Input: part model. Units: mm. Frame: model coordinates. Face numbers are marked on the shaded views. A direction names the side the tool comes from. Round coordinates to 2 decimals unless told otherwise and drop trailing zeros. Loops run counter-clockwise (first coordinate to the right, second up) from the corner with the lowest first, then second, coordinate; pieces in that order, holes last. Notation, with made-up numbers: (40, -25) - (54, -25) arc R9 cw to (54, -9) - close; hole circle Ø5 at (3, 75). An arc over 180 degrees is marked (long way). One line per question, with ' | ' between items. Start each with the question number.
Item 1: Set-up query: the marked faces 1, 2, 3 and 4. Return all of +Z, -Z, +X, -X, +Y, -Y with unobstructed straight access to the full face (end or side cutting, diameter ignored); none if empty.
Item 2: First-contact query: pin 1 (3 mm diameter, centred on x = -93, y = 44, fed in from -Z); pin 2 (7 mm diameter, centred on y = -10, z = 45, fed in from -X); pin 3 (5 mm diameter, centred on x = -86, z = 46.5, fed in from -Y). Flat tips, straight axial feed; report the tip coordinate or a pass-through.
Item 3: Section B-B, the plane y = 38. Return loops of the section in (x, z).
Item 4: Material intervals for line 1 along Z through (x, y) = (-20, -10); line 2 along Z through (x, y) = (-12.5, 12); line 3 along Y through (x, z) = (-29.25, 45), sorted ascending.
Item 5: Section C-C, the plane z = 45. Return loops of the section in (x, y).
Item 6: Section D-D, the plane x = -14. Return loops of the section in (y, z).
Item 7: Section A-A, the plane z = 75. Return loops of the section in (x, y), plus the area to 3 significant figures.
Autodesk Fusion 360 part; units mm, degrees
sketch "Sketch3" plane through (0, 0, 0) normal (0, 0, 1) x (1, 0, 0)
  line L0 (0, 0) -> (-40, 0)
  line L1 (-40, 0) -> (-40, 60)
  line L2 (-40, 60) -> (0, 60)
  line L3 (0, 60) -> (0, 0)
  line L4 (-17.9857, 0) -> (-23.9857, 0)
  line L5 (-23.9857, 0) -> (-23.9857, -20)
  line L6 (-23.9857, -20) -> (-17.9857, -20)
  line L7 (-17.9857, -20) -> (-17.9857, 0)
  line L8 (-40, 0) -> (-23.9857, -20)
  line L9 (-17.9857, 0) -> (2.0143, 0)
  line L10 (2.0143, 0) -> (2.0143, 1.9843)
  line L11 (2.0143, 1.9843) -> (2.0143, 60)
  line L12 (2.0143, 60) -> (0, 60)
  dimension "d16" = 60
  dimension "d17" = 40
  dimension "d18" = 20
  dimension "d19" = 6
  dimension "d63" = 20
extrude "Extrude1" add sketch "Sketch3" along normal blind 85 contours L0 L1 L2 L3 L4 L9 | L0 L4 L5 L6 L7 | L0 L5 L8
sketch "Sketch5" plane through (0, 0, 85) normal (0, 0, 1) x (-1, 0, 0)
  line L0 (23.9857, 20) -> (17.9857, 20)
  line L1 (17.9857, 20) -> (17.9857, 0)
  line L2 (17.9857, 0) -> (0, 0)
  line L3 (0, 0) -> (0, -60)
  line L4 (0, -60) -> (40, -60)
  line L5 (40, -60) -> (40, 0)
  line L6 (40, -60) -> (0, -60)
  line L7 (0, -6) -> (23.9857, -6)
  line L8 (23.9857, -6) -> (23.9857, 0)
  line L9 (40, 0) -> (23.9857, 20)
  line L10 (23.9857, 0) -> (23.9857, 20)
  dimension "d20" = 6
extrude "Extrude2" cut sketch "Sketch5" against normal blind 15 contours L3 L4 L5 L6 L7 L8 L9 L10
sketch "Sketch6" plane through (-40, 0, 0) normal (-1, 0, 0) x (0, -1, 0)
  line L0 (0, 70) -> (-60, 70)
  line L1 (-60, 70) -> (-60, 0)
  line L2 (-60, 0) -> (0, 0)
  line L3 (-55, 0) -> (-10, 0)
  line L4 (-10, 0) -> (-10, 60)
  line L5 (-10, 60) -> (-55, 60)
  line L6 (-55, 60) -> (-55, 0)
  line L7 (0, 0) -> (0, 70)
  dimension "d23" = 45
  dimension "d27" = 10
  dimension "d28" = 60
extrude "Extrude3" cut sketch "Sketch6" against normal blind 30 contours L2 L3 L4 L5 L6
sketch "Sketch7" plane through (0, 60, 0) normal (0, 1, 0) x (-1, 0, 0)
  line L0 (40, 70) -> (0, 70)
  line L1 (0, 70) -> (0, 0)
  line L2 (0, 0) -> (40, 0)
  line L3 (40, 0) -> (40, 70)
  line L4 (20, 70) -> (20, 10) construction
  circle A0 centre (20, 10) radius 2
  point P0 (20, 10)
  dimension "d29" = 60
  dimension "d30" = 20
  dimension "d31" = 4
extrude "Extrude4" cut sketch "Sketch7" against normal blind 57 contours A0
sketch "Sketch8" plane through (0, 55, 0) normal (0, -1, 0) x (1, 0, 0)
  circle A0 centre (-20, 10) radius 2
  line L0 (-40, 60) -> (-40, 0)
  line L1 (-40, 0) -> (-10, 0)
  line L2 (-10, 0) -> (-10, 60)
  line L3 (-10, 60) -> (-40, 60)
  line L4 (-10, 0) -> (-25, 0)
  line L5 (-25, 0) -> (-25, 10)
  line L6 (-20, 15) -> (-10, 15)
  line L7 (-10, 15) -> (-10, 0)
  arc A1 (-20, 15) -> (-25, 10) centre (-20, 10) ccw
  dimension "d34" = 5
extrude "Extrude5" add sketch "Sketch8" along normal blind 19 contours L1 L2 L4 L5 L6 L7 A1
sketch "Sketch10" plane through (0, 36, 0) normal (0, -1, 0) x (1, 0, 0)
  circle A0 centre (-20, 10) radius 2
  line L0 (-10, 15) -> (-20, 15)
  arc A1 (-20, 15) -> (-25, 10) centre (-20, 10) ccw
  line L1 (-25, 10) -> (-25, 0)
  line L2 (-25, 0) -> (-10, 0)
  line L3 (-10, 0) -> (-10, 15)
  line L4 (-20, 10) -> (-90.5618, 57.3923)
  dimension "d39" = 85
sketch "Sketch11" plane through (-40, 0, 0) normal (-1, 0, 0) x (0, -1, 0)
  line L0 (-55, 0) -> (-55, 60)
  line L1 (-55, 60) -> (-10, 60)
  line L2 (-10, 60) -> (-10, 0)
  line L3 (-10, 0) -> (0, 0)
  line L4 (0, 0) -> (0, 70)
  line L5 (0, 70) -> (-60, 70)
  line L6 (-60, 70) -> (-60, 0)
  line L7 (-60, 0) -> (-55, 0)
  line L8 (0, 70) -> (-60, 70)
  line L9 (-60, 35) -> (-55, 35)
  line L10 (-55, 60) -> (-10, 60)
  line L11 (-10, 35) -> (0, 35)
extrude "Extrude6" add sketch "Sketch11" along normal blind 60 contours L0 L1 L2 L4 L5 L6 L8 L9 L10 L11
sketch "Sketch12" plane through (0, 0, 60) normal (0, 0, -1) x (1, 0, 0)
  line L0 (-100, -55) -> (-10, -55)
  line L1 (-10, -55) -> (-10, -10)
  line L2 (-10, -10) -> (-100, -10)
  line L3 (-100, -10) -> (-100, -55)
  line L4 (-94.2104, -42.6) -> (-87.4104, -42.6)
  line L5 (-87.4104, -42.6) -> (-87.4104, -47)
  line L6 (-87.4104, -47) -> (-94.2104, -47)
  line L7 (-94.2104, -47) -> (-94.2104, -42.6)
  dimension "d71" = 6.8
  dimension "d72" = 4.4
  dimension "d73" = 8
extrude "Extrude7" add sketch "Sketch12" along normal blind 5 contours L4 L5 L6 L7
sketch "Sketch13" plane through (-94.2104, 0, 0) normal (-1, 0, 0) x (0, -1, 0)
  line L0 (-42.6, 60) -> (-47, 60)
  line L1 (-47, 60) -> (-47, 55)
  line L2 (-47, 55) -> (-42.6, 55)
  line L3 (-42.6, 55) -> (-42.6, 60)
  line L4 (-47, 58.2513) -> (-42.6, 58.2513)
  line L5 (-42.6, 58.2513) -> (-42.6, 56.9215)
  line L6 (-42.6, 56.9215) -> (-47, 56.9215)
  line L7 (-47, 56.9215) -> (-47, 58.2513)
extrude "Extrude8" cut sketch "Sketch13" against normal blind 2.5 contours L1 L3 L4 L5 L6 L7
sketch "Sketch14" plane through (0, 6, 0) normal (0, 1, 0) x (-1, 0, 0)
  line L0 (23.9857, 85) -> (0, 85)
  line L1 (0, 85) -> (0, 70) construction
  line L2 (0, 70) -> (23.9857, 70)
  line L3 (23.9857, 70) -> (23.9857, 85)
  line L4 (-2.0143, 85) -> (17.9857, 85) construction
  line L5 (17.9857, 85) -> (17.9857, 65) construction
  line L6 (17.9857, 65) -> (-2.0143, 65) construction
  line L7 (-2.0143, 65) -> (-2.0143, 85) construction
  line L8 (17.9857, 85) -> (-2.0143, 65) construction
  line L9 (-2.0143, 85) -> (17.9857, 65) construction
  point P0 (7.9857, 75)
  dimension "d68" = 6
  dimension "d69" = 20
  dimension "d70" = 20
hole "Hole3" at (-7.9857, 6, 75) direction (0, -1, 0) diameter 5 depth 10 tip angle 118
sketch "Sketch15" plane through (-23.9857, 0, 0) normal (-1, 0, 0) x (0, -1, 0)
  line L0 (20, 85) -> (-6, 85) construction
  line L1 (-6, 85) -> (-6, 70)
  line L2 (-6, 70) -> (20, 70) construction
  line L3 (20, 70) -> (20, 85) construction
  line L4 (20, 85) -> (0, 85) construction
  line L5 (0, 85) -> (0, 65) construction
  line L6 (0, 65) -> (20, 65) construction
  line L7 (20, 65) -> (20, 85) construction
  line L8 (20, 85) -> (0, 65) construction
  line L9 (0, 85) -> (20, 65) construction
  point P0 (10, 75)
  dimension "d51" = 20
  dimension "d52" = 20
hole "Hole4" at (-23.9857, -10, 75) direction (1, 0, 0) diameter 5 depth 6 tip angle 118
sketch "Sketch16" plane through (-40, 0, 0) normal (-1, 0, 0) x (0, -1, 0)
  line L0 (0, 35) -> (-10, 35)
  line L1 (-10, 35) -> (-10, 0)
  line L2 (-10, 0) -> (0, 0)
  line L3 (0, 0) -> (0, 35)
  line L4 (10, 75) -> (10, 0) construction
  point P0 (10, 15)
  point P1 (10, 45)
hole "Hole5" at (-40, -10, 15) at (-40, -10, 45) direction (1, 0, 0) diameter 5.4 depth 25 tip angle 180 counterbore diameter 8.5 counterbore depth 15
extrude "Extrude9" add 1 faces at (0, 22, 23.3333) along direction (1, 0, 0) blind 2.014
sketch "Sketch18" plane through (0, 10, 0) normal (0, 1, 0) x (-1, 0, 0)
  circle A0 centre (20, 10) radius 2
  line L0 (100, 60) -> (10, 60)
  line L1 (10, 60) -> (10, 0)
  line L2 (10, 0) -> (40, 0)
  line L3 (40, 0) -> (40, 35)
  line L4 (40, 35) -> (100, 35)
  line L5 (100, 35) -> (100, 60)
  line L6 (10, 0) -> (25, 0)
  line L7 (25, 0) -> (25, 10)
  line L8 (20, 15) -> (10, 15)
  line L9 (10, 15) -> (10, 0)
  arc A1 (25, 10) -> (20, 15) centre (20, 10) ccw
  dimension "d74" = 5
extrude "Extrude10" add sketch "Sketch18" along normal blind 3 contours L1 L2 L6 L7 L8 L9 A1
sketch "Sketch19" plane through (0, 0, 0) normal (0, -1, 0) x (1, 0, 0)
  line L0 (-40, 35) -> (-40, 70)
  line L1 (-40, 70) -> (-100, 70)
  line L2 (-100, 70) -> (-100, 35)
  line L3 (-100, 35) -> (-40, 35)
  line L4 (-75, 55) -> (-60, 55)
  line L5 (-60, 55) -> (-60, 49.5)
  line L6 (-60, 49.5) -> (-75, 49.5)
  line L7 (-75, 49.5) -> (-75, 55)
  dimension "d77" = 15
  dimension "d78" = 5.5
extrude "Extrude11" cut sketch "Sketch19" against normal blind 10 contours L4 L5 L6 L7
equation "d65 = 20 mm - 17.986 mm"
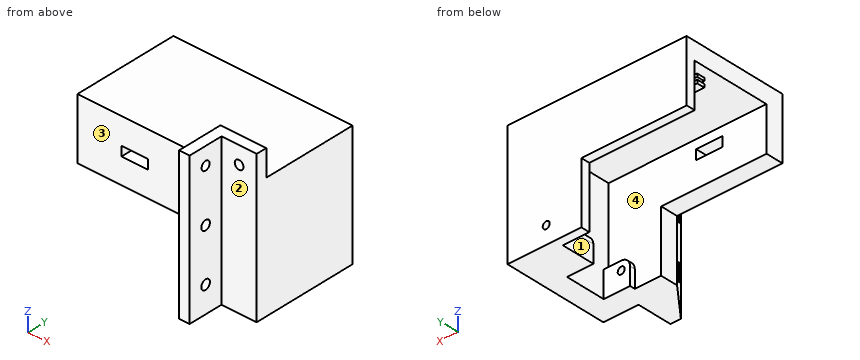
Return value:
1) face 1: -Z, -X | face 2: +Z, -Z, +X, -Y | face 3: +Z, -Z, -X, -Y | face 4: -X
2) pin 1: z = 55 | pin 2: x = -25 | pin 3: y = 0
3) outline: (-100, 60) - (-10, 60) - (-10, 15) - (-20, 15) arc R5 ccw to (-25, 10) - (-25, 0) - (2.01, 0) - (2.01, 70) - (-100, 70) - close; hole circle Ø4 at (-20, 10)
4) line 1: 0 to 12.3, 17.7 to 42.3, 47.7 to 72.5, 77.5 to 85 | line 2: 0 to 15, 60 to 70 | line 3: -5.75 to 10, 55 to 60
5) outline: (-100, 0) - (-40, 0) - (-35.4, -5.75) - (-25, -5.75) - (-25, -7.3) - (-17.99, -7.3) - (-17.99, 0) - (2.01, 0) - (2.01, 60) - (-100, 60) - (-100, 55) - (-10, 55) - (-10, 10) - (-100, 10) - close; (-28.59, -14.25) - (-23.99, -20) - (-17.99, -20) - (-17.99, -12.7) - (-25, -12.7) - (-25, -14.25) - close
6) outline: (0, 0) - (13, 0) - (13, 15) - (10, 15) - (10, 60) - (55, 60) - (55, 15) - (36, 15) - (36, 0) - (60, 0) - (60, 70) - (6, 70) - (6, 85) - (0, 85) - close
7) outline: (-23.99, -20) - (-17.99, -20) - (-17.99, -12.5) - (-23.99, -12.5) - close; (-23.99, -7.5) - (-17.99, -7.5) - (-17.99, 0) - (-10.49, 0) - (-10.49, 6) - (-23.99, 6) - close; (-5.49, 0) - (2.01, 0) - (2.01, 6) - (-5.49, 6) - close | area: 216 mm2
